Study the drawing (mm; zero at the part's minimum x, y, z) and answer. A direction names the side the tool comes from. Round coordinates to 2 decimals unless told otherwise and drop trailing zeros. Write each loop counter-clockwise with the first axis right and the second up, starting at its lowest first coordinate (ties: lowest second). Pieces come first, ordered by that corner, then holes.
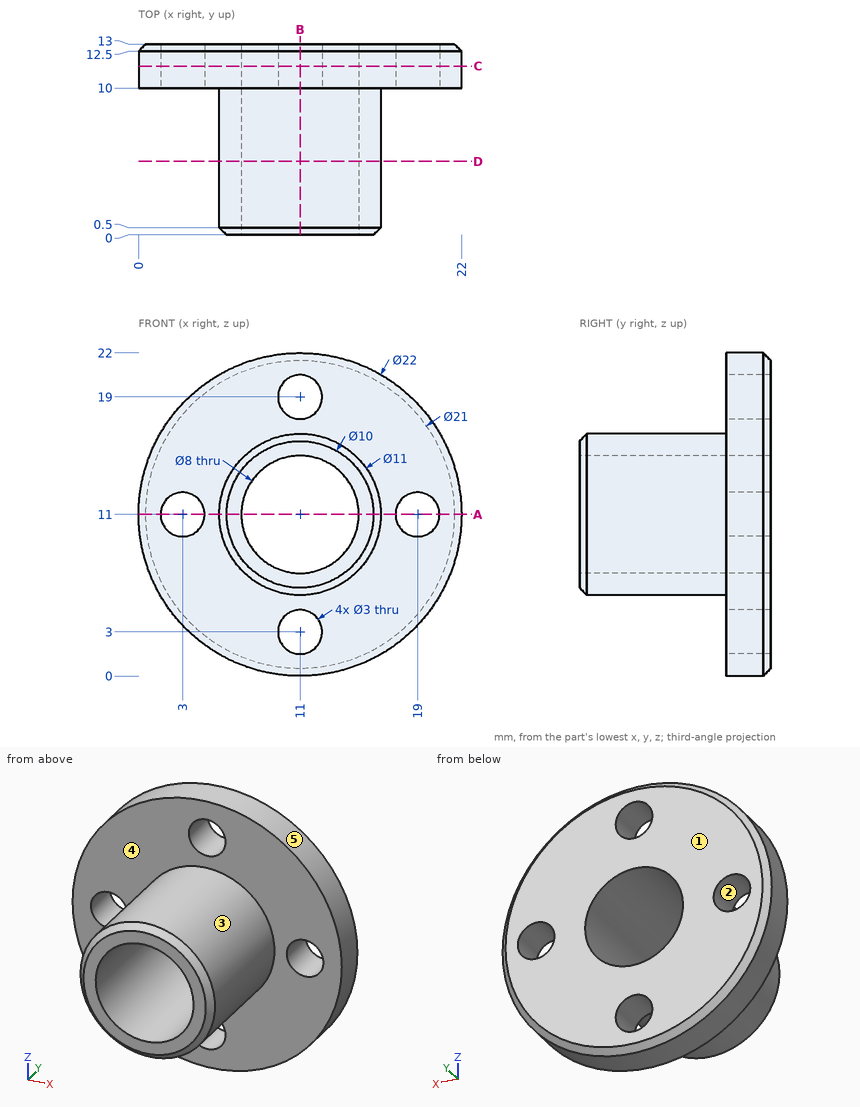
1. Straight lines are drawn through the part: line 1 along X through (y, z) = (10.65, 11); line 2 along Z through (x, y) = (11, 3.75). For each, find the intervals that lie inside material, in ascending order.
Geometry says:
line 1: x = 0 to 1.5, 4.5 to 7, 15 to 17.5, 20.5 to 22
line 2: z = 5.5 to 7, 15 to 16.5
2. Section D-D on y = 5 is taken. Determine the outline of the cut face in (x, z).
Geometry says:
outline: circle Ø11 at (11, 11); hole circle Ø8 at (11, 11)
3. For a pull along X with two mould halves and no side action, classify the marked faces 1, 2 and 3 as released by +X, released by -X, zero draft, split by the parting line, or undercut.
Geometry says:
face 1: zero draft
face 2: undercut
face 3: split by the parting line
4. Section C-C on y = 11.5 is taken. Determine the outline of the cut face in (x, z).
Geometry says:
outline: circle Ø22 at (11, 11); hole circle Ø3 at (3, 11); hole circle Ø8 at (11, 11); hole circle Ø3 at (11, 3); hole circle Ø3 at (11, 19); hole circle Ø3 at (19, 11)
5. Section A-A on z = 11 is taken. Determine the outline of the cut face in (x, y), plus the area to 3 significant figures.
Geometry says:
outline: (0, 10) - (1.5, 10) - (1.5, 13) - (0.5, 13) - (0, 12.5) - close; (4.5, 10) - (5.5, 10) - (5.5, 0.5) - (6, 0) - (7, 0) - (7, 13) - (4.5, 13) - close; (15, 0) - (16, 0) - (16.5, 0.5) - (16.5, 10) - (17.5, 10) - (17.5, 13) - (15, 13) - close; (20.5, 10) - (22, 10) - (22, 12.5) - (21.5, 13) - (20.5, 13) - close
area: 53.5 mm2
6. Section B-B on x = 11 is taken. Determine the outline of the cut face in (y, z).
Geometry says:
outline: (0, 6) - (0.5, 5.5) - (10, 5.5) - (10, 4.5) - (13, 4.5) - (13, 7) - (0, 7) - close; (0, 15) - (13, 15) - (13, 17.5) - (10, 17.5) - (10, 16.5) - (0.5, 16.5) - (0, 16) - close; (10, 0) - (12.5, 0) - (13, 0.5) - (13, 1.5) - (10, 1.5) - close; (10, 20.5) - (13, 20.5) - (13, 21.5) - (12.5, 22) - (10, 22) - close
7. A tool of negligible diameter and unlimited length cuts with its end or side. For the marked faces 4 and 5, from which of +Z, -Z, +X, -X, +Y, -Y can it reach the whole face along a straight path? Write none if from no direction.
Geometry says:
face 4: -Y
face 5: +Y, -Y
8. Given pin 1 (2.5 mm diameter, centred on x = 3, z = 11, fed in from -Y); pin 2 (3.5 mm diameter, centred on x = 19, z = 11, fed in from -Y); pin 3 (2 mm diameter, centred on x = 8, y = 5.5, fed in from +Z); pin 4 (5 mm diameter, centred on y = 5, z = 18.5, fed in from -X), each flat-ended and moving along its own axis, determine where each tip first touches the part or whether it passes through.
Geometry says:
pin 1: passes through
pin 2: stops at y = 10
pin 3: stops at z = 16.12
pin 4: stops at x = 8.71
